Read the model definition and answer for the solid it produces. Units are mm, in the model's axes. Face numbers are marked on the shaded views. A direction names the side the tool comes from. Coordinates: 2 decimals unless noted, no trailing zeros. Order: outer loops, then holes, each group sorted by start corner. A loop starts at its lowest first (then second) coordinate and runs counter-clockwise, first axis right, second up. Notation, with made-up numbers: (84.5, -7.75) - (141.5, -7.75) arc R22 cw to (141.5, 10.25) - close; hole circle Ø6 at (58, 31). An arc over 180 degrees is marked (long way). Use one line per item in the form item = value. Start each with the question number.
from build123d import *

# Parameters (mm, degrees)
CYLINDER_R           = 15
CYLINDER_DEPTH       = 100
CYLINDER_PITCH_ANGLE = 90
BOX005_W             = 100
BOX005_H             = 30
BOX005_DEPTH         = 30
BOX004_W             = 40
BOX004_H             = 40
BOX004_DEPTH         = 120
BOX004_ROLL_ANGLE    = -5.2
BOX003_W             = 40
BOX003_H             = 40
BOX003_DEPTH         = 120
BOX003_ROLL_ANGLE    = 5.2
BOX001_W             = 19
BOX001_H             = 100
BOX001_DEPTH         = 110
BOX001_PITCH_ANGLE   = 8.4
BOX_W                = 25
BOX_H                = 80
BOX_DEPTH            = 100
THICKNESS_T          = 1


with BuildPart() as cylinder:
    # Cylinder → Cylinder (new body)
    with BuildSketch(Plane.XY):
        Circle(CYLINDER_R)
    extrude(amount=CYLINDER_DEPTH)


with BuildPart() as cylinder_1:
    # Cylinder pitch: moved
    add(cylinder.part.rotate(Axis((0, 0, 0), (0, 1, 0)), CYLINDER_PITCH_ANGLE))


with BuildPart() as cylinder_2:
    # Cylinder placement: moved
    add(cylinder_1.part.moved(Location((0, 40, 70))))


with BuildPart() as fusion:
    # Box005 → Box005 (new body)
    with BuildSketch(Plane(origin=(0, 25, 70), x_dir=(1, 0, 0), z_dir=(0, 0, 1))):
        with Locations((50, 15)):
            Rectangle(BOX005_W, BOX005_H)
    extrude(amount=BOX005_DEPTH)

    # Fusion: union Cylinder
    add(cylinder_2.part)


with BuildPart() as cube002:
    # Box004 → Box004 (new body)
    with BuildSketch(Plane.XY):
        with Locations((20, 20)):
            Rectangle(BOX004_W, BOX004_H)
    extrude(amount=BOX004_DEPTH)


with BuildPart() as cube002_1:
    # Box004 roll: moved
    add(cube002.part.rotate(Axis((0, 0, 0), (1, 0, 0)), BOX004_ROLL_ANGLE))


with BuildPart() as cube002_2:
    # Box004 placement: moved
    add(cube002_1.part.moved(Location((0, 70, -4))))


with BuildPart() as cube003:
    # Box003 → Box003 (new body)
    with BuildSketch(Plane.XY):
        with Locations((20, 20)):
            Rectangle(BOX003_W, BOX003_H)
    extrude(amount=BOX003_DEPTH)


with BuildPart() as cube003_1:
    # Box003 roll: moved
    add(cube003.part.rotate(Axis((0, 0, 0), (1, 0, 0)), BOX003_ROLL_ANGLE))


with BuildPart() as cube003_2:
    # Box003 placement: moved
    add(cube003_1.part.moved(Location((0, -30, -4))))


with BuildPart() as cube001:
    # Box001 → Box001 (new body)
    with BuildSketch(Plane.XY):
        with Locations((9.5, 50)):
            Rectangle(BOX001_W, BOX001_H)
    extrude(amount=BOX001_DEPTH)


with BuildPart() as cube001_1:
    # Box001 pitch: moved
    add(cube001.part.rotate(Axis((0, 0, 0), (0, 1, 0)), BOX001_PITCH_ANGLE))


with BuildPart() as cube001_2:
    # Box001 placement: moved
    add(cube001_1.part.moved(Location((10, 0, 0))))


with BuildPart() as thickness:
    # Box → Box (new body)
    with BuildSketch(Plane.XY):
        with Locations((12.5, 40)):
            Rectangle(BOX_W, BOX_H)
    extrude(amount=BOX_DEPTH)

    # Cut: cut Cube001
    add(cube001_2.part, mode=Mode.SUBTRACT)

    # Cut001: cut Cube003
    add(cube003_2.part, mode=Mode.SUBTRACT)

    # Cut002: cut Cube002
    add(cube002_2.part, mode=Mode.SUBTRACT)

    # Cut003: cut Fusion
    add(fusion.part, mode=Mode.SUBTRACT)

    # Thickness
    thickness_openings = [thickness.faces().sort_by_distance(p)[0] for p in [
        (0, 40.100786, 46.297736),
    ]]
    offset(amount=THICKNESS_T, openings=thickness_openings)


solid = thickness.part
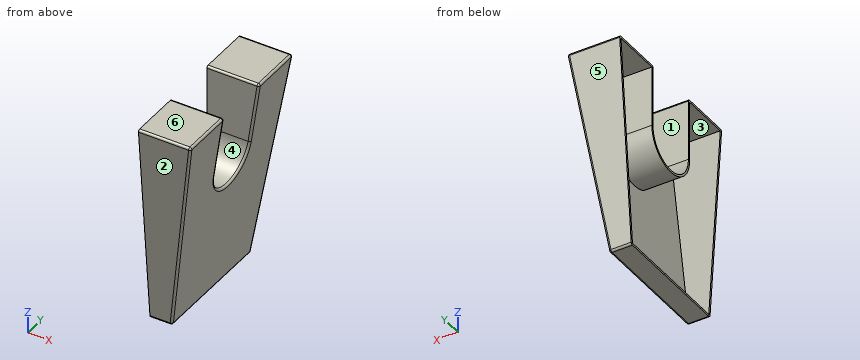
Q1. Which of the six approach directions +Z, -Z, +X, -X, +Y, -Y give full straight-line access (tool end or side, diameter ignored) to the marked faces 1, 2 and 3?
Q2. Consider probe 1 along Z at (x, y) = (7.5, 63); probe 2 along Y at (x, z) = (20.25, 81.5); probe 3 along Y at (x, z) = (5.5, 83). Determine where each line is inside the solid, lowest interval first.
Q3. Given P1, Ø10, axis at x = 4, z = 36, coming from the +Y side; P2, Ø6, axis at y = 20.5, z = 80.5, coming from the +X side; P3, Ø6, axis at y = 34.5, z = 52, coming from the +X side; P4, Ø1, axis at x = 20.5, y = 41, coming from the +Z side, each flat-ended and moving along its own axis, determine where each tip first touches the part or whether it passes through.
Q4. For a pull along Y with two mould halves and no side action, classify the marked faces 4, 5 and 6 as +Y half, -Y half, draft (parallel to the pull), parting line (faces both ways), or undercut.
Q5. A cutting plane is placed at A-A (y = 66.5). Give the vertices of the cut face in (x, z), then the cut area to 3 significant figures.
Result sheet:
q1.face_1 = +Z, +X, -X
q1.face_2 = -Z, +X, -X, -Y
q1.face_3 = -X
q2.probe_1 = -1 to 0, 100 to 101
q2.probe_2 = 1.38 to 2.38, 25 to 26, 54 to 55, 77.78 to 78.79
q2.probe_3 = 1.24 to 2.25, 25 to 26, 54 to 55, 77.92 to 78.92
q3.P1 = 75.1
q3.P2 = 23.34
q3.P3 = 19.13
q3.P4 = through
q4.face_4 = undercut
q4.face_5 = +Y half
q4.face_6 = draft
q5.outline = (0, -1) - (10, -1) arc R1 ccw to (10.99, -0.15) - (25.76, 99.85) arc R1 ccw to (24.77, 101) - (0, 101) - (0, 100) - (24.77, 100) - (10, 0) - (0, 0) - close
q5.area = 137 mm^2
